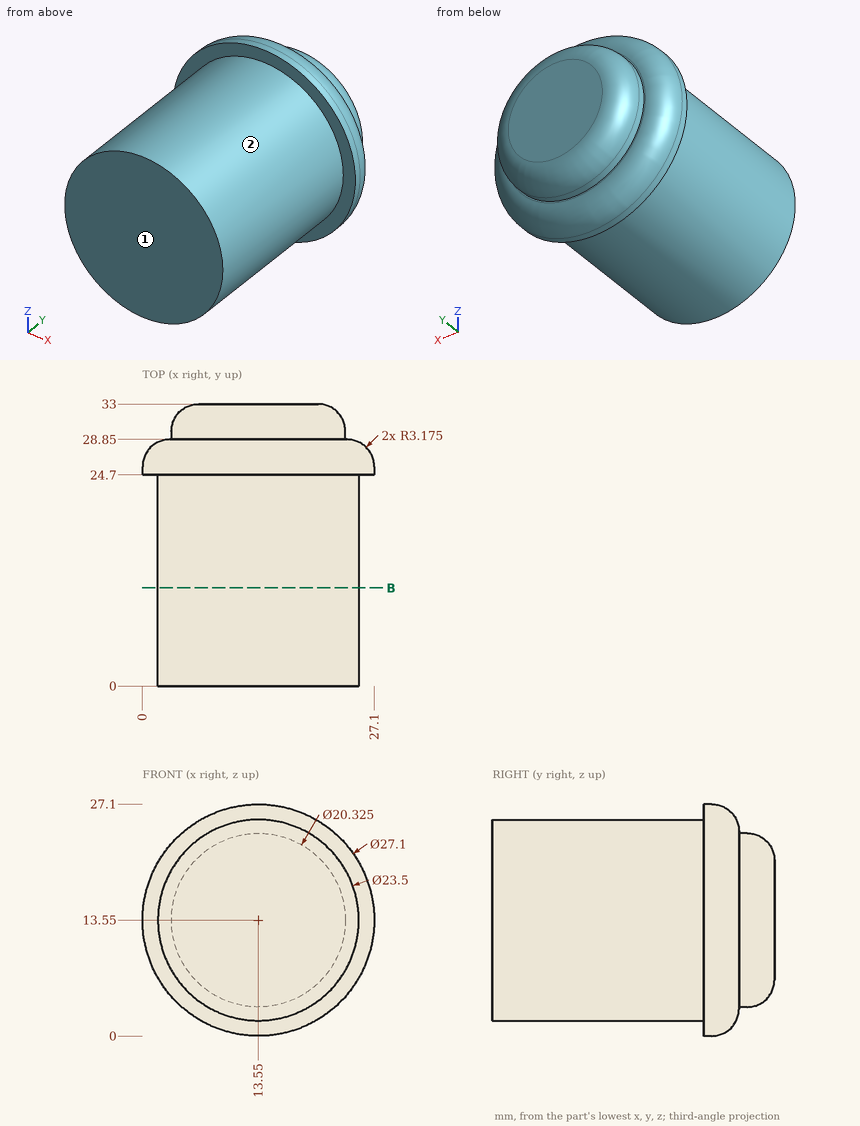
Could you check a few things on this drawing? It's one solid part, dimensions in mm from its lowest x, y, z. A direction names the side the tool comes from. Coordinates: 2 decimals unless noted, no trailing zeros. Order: outer loops, then holes, each group sorted by start corner. A loop starts at its lowest first (then second) coordinate and runs counter-clockwise, first axis right, second up. Notation, with made-up numbers: M 32,72.25 L 73,72.25 A8 cw 73,83.25 Z; hole C 46,87 d5. An arc over 180 degrees is marked long. Use one line per item in the form item = value. Start each with the question number.
1. Please list where these lines run through material, in increasing order: line 1 (Y direction, x = 7, z = 16.5); line 2 (Y direction, x = 4.5, z = 18.5); line 3 (X direction, y = 2.5, z = 4).
2. On a 3-axis mill with a long thin cutter (end or side, diameter ignored), from which of +Z, -Z, +X, -X, +Y, -Y can I reach the whole of each face in a straight line? I mean the marked faces 1 and 2. Say none if no direction works.
3. Suppose I cut it at B-B on y = 11.5. Write out the boundary of the cut face in (x, z).
4. For pin 1 (12 mm diameter, centred on x = 9, y = 5.5, fed in from -Z); pin 2 (5 mm diameter, centred on x = 18, y = 7.5, fed in from +Z); pin 3 (2 mm diameter, centred on x = 4.5, y = 22.5, fed in from -Z); pin 4 (10 mm diameter, centred on x = 20.5, z = 10.5, fed in from -Y), each with a flat end and sliding along its axis, tell me the tip position at first contact or that it passes through.
Geometry says:
q1.line_1 = 0 to 32.99
q1.line_2 = 0 to 28.85
q1.line_3 = 6.7 to 20.4
q2.face_1 = +Z, -Z, +X, -X, -Y
q2.face_2 = -Y
q3.outline = C 13.55,13.55 d23.5
q4.pin_1 = 1.8
q4.pin_2 = 25.14
q4.pin_3 = 4.99
q4.pin_4 = 0
